Check sheet for the modelled part. Datum: model origin and axes. Units: mm. A direction names the side the tool comes from. Coordinates: 2 decimals unless noted, no trailing zeros. Loops run counter-clockwise (first coordinate to the right, second up) from the corner with the lowest first, then second, coordinate; pieces in that order, holes last.
Autodesk Inventor part; units mm, degrees
ref_plane "YZ-Ebene" through (0, 0, 0) normal (1, 0, 0) x (0, 1, 0)
ref_plane "XY-Ebene" through (0, 0, 0) normal (0, 0, 1) x (1, 0, 0)
sketch "Skizze1" plane through (0, 0, 0) normal (0, 0, 1) x (1, 0, 0)
  line L0 (-7, 0) -> (42, 0)
  line L1 (0, -1.8) -> (0, 10.8)
  line L2 (0, 2.8) -> (20, 2.8)
  line L3 (20, 2.8) -> (20, 2.25)
  line L4 (20, 2.25) -> (35, 2.25)
  line L5 (35, 2.25) -> (35, 3.7)
  line L6 (35, 3.7) -> (28.2, 4.5)
  line L7 (28.2, 4.5) -> (3, 4.5)
  line L8 (3, 4.5) -> (3, 9)
  line L9 (3, 9) -> (0, 9)
  line L10 (0, 9) -> (0, 2.8)
  point P0 (0, 0)
  dimension "d0" = 35
  dimension "d1" = 9
  dimension "d2" = 4.5
  dimension "d3" = 2.8
  dimension "d4" = 2.25
  dimension "d5" = 3.7
  dimension "d6" = 3
  dimension "d7" = 6.8
  dimension "d8" = 20
revolve "Umdrehung1" add sketch "Skizze1" angle 360 about axis through (-10, 0, 0) along (1, 0, 0)
chamfer "Fase1" distance 0.5 distance2 0.5 1 edges at (35, -2.25, 0) measured on face at (30, 2.2209, -0.3609)
ref_plane "Arbeitsebene1" through (15.6, -4.5, 0) normal (0, 1, 0) x (-1, 0, 0)
sketch "Skizze2" plane through (15.6, -4.5, 0) normal (0, 1, 0) x (-1, 0, 0)
  line L0 (15.6, 9) -> (15.6, -9)
  line L1 (6.6, 2.4) -> (-1.4, 2.4)
  line L2 (-2.4, 1.4) -> (-2.4, -1.4)
  line L3 (-1.4, -2.4) -> (6.6, -2.4)
  line L4 (7.6, -1.4) -> (7.6, 1.4)
  arc A0 (7.6, 1.4) -> (6.6, 2.4) centre (6.6, 1.4) ccw
  arc A1 (-1.4, 2.4) -> (-2.4, 1.4) centre (-1.4, 1.4) ccw
  arc A2 (-2.4, -1.4) -> (-1.4, -2.4) centre (-1.4, -1.4) ccw
  arc A3 (6.6, -2.4) -> (7.6, -1.4) centre (6.6, -1.4) ccw
  line L5 (12.6, 4.5) -> (12.6, -4.5)
  line L6 (-12.6, 4.5) -> (-12.6, -4.5)
  line L7 (12.6, 4.5) -> (12.6, -4.5)
  line L8 (-4.4, -2.8) -> (15.6, -2.8)
  point P0 (15.6, 0)
  point P1 (-2.4, -2.4)
  point P2 (-2.4, 2.4)
  point P3 (7.6, -2.4)
  dimension "d13" = 10
  dimension "d14" = 8
  dimension "d15" = 4.8
  dimension "d16" = 1
extrude "Extrusion1" cut sketch "Skizze2" along normal up to next
sketch "Skizze3" plane through (0, 0, 0) normal (-1, 0, 0) x (0, 0, 1)
  circle A0 centre (0, 0) radius 2.8
  circle A1 centre (0, 0) radius 9
  circle A2 centre (-4.1012, 4.1012) radius 1.8
  line L0 (0, -12.6) -> (0, 12.6)
  line L1 (0, 0) -> (-4.1012, 4.1012) construction
  dimension "d19" = 3.6
  dimension "d23" = 5.8
  dimension "d24" = 45
extrude "Extrusion2" add sketch "Skizze3" along normal blind 4 contours A2
sketch "Skizze4" plane through (0, 0, 0) normal (-1, 0, 0) x (0, 0, 1)
  circle A0 centre (-4.1012, 4.1012) radius 1.8
  circle A1 centre (0, 0) radius 9
  line L0 (0, 0) -> (-4.1012, 4.1012) construction
  arc A2 (0, 6.364) -> (-6.364, 6.364) centre (-3.182, 3.182) ccw
  line L1 (0, 6.364) -> (2.1213, 4.2426)
  arc A3 (2.1213, 4.2426) -> (6.5007, 4.2102) centre (4.3275, 6.4488) ccw
  arc A4 (8.097, 3.9293) -> (6.5007, 4.2102) centre (7.1973, 3.4927) ccw
  dimension "d28" = 9
  dimension "d32" = 4.5
  dimension "d33" = 3.12
  dimension "d34" = 1
  dimension "d36" = 3
extrude "Extrusion3" cut sketch "Skizze4" against normal through all contours A4 A3 L1 A2 A1 picked at (1.838, 6.3142)
ref_plane "Arbeitsebene2" through (0, 0, 0) normal (0, 0.7071, 0.7071) x (1, 0, 0)
mirror "Spiegeln1" about plane through (0, 0, 0) normal (0, 1, 0) of "Extrusion3"
thread "Gewinde1"
ref_plane "Arbeitsebene3" through (0, 0, 0) normal (0, 0.7071, -0.7071) x (1, 0, 0)
properties part number "Kurbelwelle_ra8846s" material "Stahl"
1) Mould release check, pull along X, two halves, no side actions. Record for faces 1 (the flat face through (13, -3, 2.4)), 2 (the cylindrical face through (8.285, -2.879, -2.099)), 3 (the flat face through (0, 0, -4)), 4 (the cylindrical face through (27.35, -0.29, 2.23)): +X half, -X half, draft (parallel to the pull), parting line (faces both ways), or undercut.
Answer sheet:
face 1: undercut
face 2: undercut
face 3: -X half
face 4: draft
2) Set-up check for faces 5 (the flat face through (8, -3, 0)), 6 (the flat face through (3, 3, -4)), 7 (the cylindrical face through (1.48, 7.68, -3.13)): record each of +Z, -Z, +X, -X, +Y, -Y from which the full face is reachable in a straight line by a thin tool's end or side.
Answer sheet:
face 5: -Y
face 6: +X
face 7: +X, -X, +Y
3) Depth check by flat-ended pin: pin 1 (0.6 mm diameter, centred on y = -4, z = 0.5, fed in from -X); pin 2 (0.7 mm diameter, centred on x = 11.5, y = -2.5, fed in from +Z); pin 3 (5 mm diameter, centred on y = 0, z = 0, fed in from +X). Enter the tip coordinate at first touch or a pass-through.
Answer sheet:
pin 1: stops at x = 0
pin 2: stops at z = 3.95
pin 3: stops at x = 34.75
4) Scan lines: line 1 (Y direction, x = 5.75, z = 0); line 2 (Z direction, x = 25.5, y = 0). Record each from-to range of solid material in increasing order.
Answer sheet:
line 1: y = -4.5 to -2.8, 2.8 to 4.5
line 2: z = -4.5 to -2.25, 2.25 to 4.5
5) Section check B-B on x = 2.5. Enter the section's corners in (y, z).
Answer sheet:
outline: (-6.36, -6.36) arc R9 ccw to (6.36, -6.36) arc R4.5 ccw to (6.36, 0) - (4.24, 2.12) arc R3.12 cw to (4.21, 6.5) arc R1 ccw to (3.93, 8.1) arc R9 ccw to (-3.93, 8.1) arc R1 ccw to (-4.21, 6.5) arc R3.12 cw to (-4.24, 2.12) - (-6.36, 0) arc R4.5 ccw to start; hole circle Ø5.6 at (0, 0)
6) Section check A-A on y = 0. Enter the section's corners in (x, z), plus the area to 3 significant figures.
Answer sheet:
outline: (0, -9) - (3, -9) - (3, -4.5) - (28.2, -4.5) - (35, -3.7) - (35, -2.75) - (34.5, -2.25) - (20, -2.25) - (20, -2.8) - (0, -2.8) - close; (0, 2.8) - (20, 2.8) - (20, 2.25) - (34.5, 2.25) - (35, 2.75) - (35, 3.7) - (28.2, 4.5) - (3, 4.5) - (3, 9) - (0, 9) - close
area: 157 mm2
7) Section check D-D on x = 14. Enter the section's corners in (y, z).
Answer sheet:
outline: (-3.81, -2.4) arc R4.5 ccw (long way) to (-3.81, 2.4) - (-1.44, 2.4) arc R2.8 cw (long way) to (-1.44, -2.4) - close
8) Section check C-C on z = -5.5. Enter the section's corners in (x, y), plus the area to 3 significant figures.
Answer sheet:
outline: (-4, 2.97) - (0, 2.97) - (0, -7.04) - (3, -7.04) - (3, 7.04) - (0, 7.04) - (0, 5.23) - (-4, 5.23) - close
area: 51.3 mm2
